Work out the finished part from the listing and answer in its coordinate system (mm). A direction names the side the tool comes from. Give positions to 0.01 mm unless a question says otherwise; leave off trailing zeros. Loops run counter-clockwise (first coordinate to the right, second up) from the corner with the lowest first, then second, coordinate; pieces in that order, holes last. Notation, with made-up numbers: M 37,-30.75 L 95,-30.75 A21 ccw 95,2.25 Z; hole C -32,72 d4. An arc over 180 degrees is marked long. Answer in a Markdown table with one row per item. Add a question column.
from build123d import *

# Parameters (mm, degrees)
EXTRUDE_1_DEPTH     = 14
SKETCH_5_R          = 1.5
CUT_EXTRUDE_1_DEPTH = 14
SKETCH_6_R          = 1
CUT_EXTRUDE_2_DEPTH = 14


with BuildPart() as part:
    # 草图1 → 凸台-拉伸1 (new body)
    with BuildSketch(Plane(origin=(0, 0, 0), x_dir=(0, 0, -1), z_dir=(1, 0, 0))):
        Polygon((0, 0), (10, 0), (10, 30), (-7, 30), (-7, 28), (8, 28), (8, 2), (0, 2), align=None)
    extrude(amount=EXTRUDE_1_DEPTH)

    # 草图5 → 切除-拉伸1 (cut)
    with BuildSketch(Plane(origin=(0, 0, -10), x_dir=(-1, 0, 0), z_dir=(0, 0, -1))):
        with Locations((-7.028963354, 21.5)):
            Circle(SKETCH_5_R)
        with Locations((-7, 4.5)):
            Circle(SKETCH_5_R)
    extrude(amount=-CUT_EXTRUDE_1_DEPTH, mode=Mode.SUBTRACT)

    # 草图6 → 切除-拉伸2 (cut)
    with BuildSketch(Plane(origin=(0, 30, 0), x_dir=(1, 0, 0), z_dir=(0, 1, 0))):
        with Locations(Location((4, 0, 0), (0, 0, 270))):
            Circle(SKETCH_6_R)
        with Locations(Location((9, 0, 0), (0, 0, 270))):
            Circle(SKETCH_6_R)
    extrude(amount=-CUT_EXTRUDE_2_DEPTH, mode=Mode.SUBTRACT)


solid = part.part
(1) Which of the six approach directions +Z, -Z, +X, -X, +Y, -Y give full straight-line access (tool end or side, diameter ignored) to faces 4 (the face through (10, 29, 0)), 5 (the face through (7, 1, 0)), 6 (the face through (7, 15, -8)), 7 (the face through (7, 15, -10)), 8 (the face through (8.5, 4.57, -9.01))?
(2) Section C-C, the plane y = 4.5 is taken. Determine the outline of the cut face in (x, z).
(3) Section D-D, the plane x = 1.75 is taken. Determine the outline of the cut face in (y, z), and give its area (3 significant figures).
(4) Consider line 1 along X through (y, z) = (29.05, 0); line 2 along Y through (x, z) = (9.75, -1.75); line 3 along Z through (x, y) = (11, 25). Determine where each line is inside the solid, lowest interval first. Write a range as from..to.
(5) Section A-A, the plane x = 4 is taken. Determine the outline of the cut face in (y, z), and give its area (3 significant figures).
(6) The mould has two halves that part along Z. Classify faces 1 (the face through (5, 29, 0)), 2 (the face through (7, 29, 7)), 3 (the face through (7, 30, -2)): pulls with the +Z half, pulls with the -Z half, needs draft (parallel to the pull), parting line crosses it, or undercut.
(7) Section B-B, the plane z = -2.75 is taken. Determine the outline of the cut face in (x, y), and give its area (3 significant figures).
(8) Each of these flat-tipped pins is pushed along its axis until it touches: P1, Ø5, axis at x = 4, y = 19, coming from the +Z side; P2, Ø2.5, axis at x = 7, y = 4.5, coming from the +Z side; P3, Ø0.6, axis at x = 6.5, y = 1, coming from the +Z side. Where does it stop, or does it pass through?
Numbers:
| question | item | result |
|---|---|---|
| 1 | face 4 | +Y |
| 1 | face 5 | +Z, +X, -X, -Y |
| 1 | face 6 | +Z, +X, -X |
| 1 | face 7 | -Z, +X, -X, +Y, -Y |
| 1 | face 8 | +Z, -Z |
| 2 | outline | M 0,-10 L 5.5,-10 L 5.5,-8 L 0,-8 Z; M 8.5,-10 L 14,-10 L 14,-8 L 8.5,-8 Z |
| 3 | outline | M 0,-10 L 30,-10 L 30,7 L 28,7 L 28,-8 L 2,-8 L 2,0 L 0,0 Z |
| 3 | area | 106 mm² |
| 4 | line 1 | x = 0..3, 5..8, 10..14 |
| 4 | line 2 | y = 0..2, 28..30 |
| 4 | line 3 | z = -10..-8 |
| 5 | outline | M 0,-10 L 30,-10 L 30,-1 L 28,-1 L 28,-8 L 2,-8 L 2,0 L 0,0 Z; M 28,1 L 30,1 L 30,7 L 28,7 Z |
| 5 | area | 102 mm² |
| 6 | face 1 | undercut |
| 6 | face 2 | pulls with the +Z half |
| 6 | face 3 | needs draft |
| 7 | outline | M 0,0 L 14,0 L 14,2 L 0,2 Z; M 0,28 L 14,28 L 14,30 L 0,30 Z |
| 7 | area | 56.0 mm² |
| 8 | P1 | stops at z = -8 |
| 8 | P2 | passes through |
| 8 | P3 | stops at z = 0 |
